```python
from build123d import *

# Parameters (mm, degrees)
SKETCH1_R           = 11.5
BOSS_EXTRUDE1_DEPTH = 10
SKETCH2_R           = 8.5
CUT_EXTRUDE2_DEPTH  = 10
SKETCH4_R           = 4
BOSS_EXTRUDE2_DEPTH = 10
BOSS_EXTRUDE3_START = 10
BOSS_EXTRUDE3_DEPTH = 10
CIRPATTERN1_COUNT   = 5
SKETCH7_R           = 1.45
CUT_EXTRUDE3_DEPTH  = 10
SKETCH8_R           = 1.75
BOSS_EXTRUDE4_DEPTH = 2
CUT_EXTRUDE4_START  = -2
SKETCH9_R           = 1.45
CUT_EXTRUDE4_DEPTH  = 2
FILLET1_R           = 2.25


with BuildPart() as part:
    # Sketch1 → Boss-Extrude1 (new body)
    with BuildSketch(Plane.XY):
        Circle(SKETCH1_R)
    extrude(amount=BOSS_EXTRUDE1_DEPTH)

    # Sketch2 → Cut-Extrude2 (cut)
    with BuildSketch(Plane.XY.offset(10)):
        Circle(SKETCH2_R)
    extrude(amount=-CUT_EXTRUDE2_DEPTH, mode=Mode.SUBTRACT)



with BuildPart() as body_2:
    # Sketch4 → Boss-Extrude2 (new body)
    with BuildSketch(Plane.XY):
        Circle(SKETCH4_R)
    extrude(amount=BOSS_EXTRUDE2_DEPTH)


with BuildPart() as part_1:
    add(part.part)

    add(body_2.part)  # Boss-Extrude3 merges body 2
    # Sketch6 → Boss-Extrude3 (add)
    with BuildSketch(Plane.XY.offset(BOSS_EXTRUDE3_START)):
        with BuildLine():
            Line((-1.114437127, 3.841618134), (-2.368178894, 8.163438536))
            ThreePointArc((-2.368178894, 8.163438536), (-0.122551325, 8.499116494), (2.131821106, 8.228325393))
            Line((2.131821106, 8.228325393), (0.940332104, 3.887901173))
            ThreePointArc((0.940332104, 3.887901173), (-0.090075911, 3.998985663), (-1.114437127, 3.841618134))
        make_face()
    boss_extrude3 = extrude(amount=-BOSS_EXTRUDE3_DEPTH)

    # CirPattern1: Boss-Extrude3 ×5 about axis
    cirpattern1_axis = Axis((0, 0, 0), (0, 0, 1))
    for i in range(1, CIRPATTERN1_COUNT):
        add(boss_extrude3.rotate(cirpattern1_axis, i * 360 / CIRPATTERN1_COUNT))

    # Sketch7 → Cut-Extrude3 (cut)
    with BuildSketch(Plane.XY.offset(10)):
        Circle(SKETCH7_R)
    extrude(amount=-CUT_EXTRUDE3_DEPTH, mode=Mode.SUBTRACT)

    # Sketch8 → Boss-Extrude4 (add)
    with BuildSketch(Plane(origin=(0, 0, 0), x_dir=(-1, 0, 0), z_dir=(0, 0, -1))):
        with Locations(Location((0, 0, 0), (0, 0, 180))):
            Circle(SKETCH8_R)
    extrude(amount=BOSS_EXTRUDE4_DEPTH)

    # Sketch9 → Cut-Extrude4 (cut)
    with BuildSketch(Plane(origin=(0, 0, -2), x_dir=(-1, 0, 0), z_dir=(0, 0, -1)).offset(CUT_EXTRUDE4_START)):
        with Locations(Location((0, 0, 0), (0, 0, 180))):
            Circle(SKETCH9_R)
    extrude(amount=CUT_EXTRUDE4_DEPTH, mode=Mode.SUBTRACT)

    # Fillet1
    # the kernel refuses this fillet: 2.25 mm, written as the material it adds along each edge
    with BuildSketch(Plane(origin=(0, 0, 0), x_dir=(1, 0, 0), z_dir=(0, 1, 0))) as fillet1_piece_1:
        with BuildLine():
            CenterArc((3.986067977, 2.25), FILLET1_R, 186.379370208, 83.620629792)
            Line((1.75, 2), (1.70527864, 1.995))
            ThreePointArc((1.70527864, 1.995), (1.705, 1), (1.705, 0))
            Line((1.705, 0), (1.75, -0.045))
            Line((1.75, -0.045), (3.986067977, -0.045))
            Line((3.986067977, -0.045), (3.986067977, 0))
        make_face()
    revolve(axis=Axis((0, 0, 0), (0, 0, -1)))


solid = part_1.part
```
Can you work these out from the model? Positions are in its coordinate system, mm. A direction names the side the tool comes from. Coordinates: 2 decimals unless noted, no trailing zeros. Loops run counter-clockwise (first coordinate to the right, second up) from the corner with the lowest first, then second, coordinate; pieces in that order, holes last. Notation, with made-up numbers: (73.25, -7) - (108.25, -7) arc R9 cw to (108.25, 1) - close; hole circle Ø3 at (-12.75, 56.25). An arc over 180 degrees is marked (long way). Answer as CSV lines item,"result". Start each with the question number.
1) Suppose I cut it at B-B (z = 3). Please give me the cut outline in (x, y), plus the area to 3 significant figures.
2) For pin 1 (3 mm diameter, centred on y = -4.5, z = 3.5, fed in from +X); pin 2 (3 mm diameter, centred on x = -7, z = 5, fed in from -Y); pin 3 (5 mm diameter, centred on y = 3.5, z = 3, fed in from -X), each with a flat end and sliding along its axis, tell me the tip position at first contact or that it passes through.
3) Thinking about a two-plate mould opening in Y: for faces 1 (the flat face through (0, -2, 10)), 2 (the cylindrical face through (-1.5, 11.4, 4.9)), 3 (the cylindrical face through (2.29, 3.28, 4.93)), which applies, pulls with the +Y half, pulls with the -Y half, needs draft (parallel to the pull), parting line crosses it, or undercut?
4) Suppose I cut it at C-C (z = -0.5). Please give me the cut outline in (x, y), plus the area to 3 significant figures.
5) Suppose I cut it at A-A (x = 0). Count the separate pieces of the cut face and the enclosed holes in it, plus the area to 3 significant figures.
6) I need wall thicknesses on line 1 (Y direction, x = 0, z = 7.5); line 2 (X direction, y = 4.75, z = 4); line 3 (Y direction, x = 5.25, z = 6.5). Which ranges of each line are inside material? Lowest first, please. Write a range as from..to.
7) Which directions (+Z, -Z, +X, -X, +Y, -Y) give clear straight access to the entire face, cutting with the end or side of a thin tool? Please do faces 4 (the flat face through (2.4, -5, 0)), 5 (the cylindrical face through (4.932, 6.923, 5.07)).
Check result:
1,outline,"circle Ø23 at (0, 0); hole (-8.5, 0.27) arc R8.5 ccw to (-6.56, -5.4) - (-3.05, -2.59) arc R4 cw to (-4, 0.13) - close; hole (-7.17, 4.57) - (-3.41, 2.1) arc R4 cw to (-1.11, 3.84) - (-2.37, 8.16) arc R8.5 ccw to start; hole (-2.88, -8) arc R8.5 ccw to (3.11, -7.91) - (1.52, -3.7) arc R4 cw to (-1.36, -3.76) - close; hole circle Ø2.9 at (0, 0); hole (0.94, 3.89) arc R4 cw to (3.31, 2.25) - (7.03, 4.77) arc R8.5 ccw to (2.13, 8.23) - close; hole (3.16, -2.45) - (6.71, -5.21) arc R8.5 ccw to (8.48, 0.52) - (3.99, 0.31) arc R4 cw to start"
1,area,"307 mm²"
2,pin 1,"stops at x = 11.1"
2,pin 2,"stops at y = -10.1"
2,pin 3,"stops at x = -11.46"
3,face 1,"needs draft"
3,face 2,"parting line crosses it"
3,face 3,"undercut"
4,outline,"circle Ø5.14 at (0, 0); hole circle Ø2.9 at (0, 0)"
4,area,"14.2 mm²"
5,separate pieces,"3"
5,enclosed holes,"0"
5,area,"159 mm²"
6,line 1,"y = -11.5..-8.5, -4..-1.45, 1.45..11.5"
6,line 2,"x = -10.47..-7.05, -1.38..1.18, 7..10.47"
6,line 3,"y = -10.23..-4.08, 0.37..3.56, 6.68..10.23"
7,face 4,"-Z"
7,face 5,"+Z, -Z"
